from build123d import *

# Parameters (mm, degrees)
SKETCH1_R           = 15.875
BOSS_EXTRUDE1_DEPTH = 12.7
CUT_EXTRUDE1_DEPTH  = 13.7
SKETCH3_R           = 15.875
BOSS_EXTRUDE2_DEPTH = 2.54
SKETCH4_R           = 15.08125
CUT_EXTRUDE2_DEPTH  = 2.54


with BuildPart() as part:
    # Sketch1 → Boss-Extrude1 (new body)
    with BuildSketch(Plane(origin=(0, 0, 0), x_dir=(1, 0, 0), z_dir=(0, 1, 0))):
        Circle(SKETCH1_R)
    extrude(amount=BOSS_EXTRUDE1_DEPTH)

    # Sketch2 → Cut-Extrude1 (cut, through all)
    with BuildSketch(Plane(origin=(0, 12.7, 0), x_dir=(1, 0, 0), z_dir=(0, 1, 0))):
        Polygon((-9.38920922, -5.728023239), (0.266009029, -10.995305325), (9.655218248, -5.267282086), (9.38920922, 5.728023239), (-0.266009029, 10.995305325), (-9.655218248, 5.267282086), align=None)
        Polygon((-5.267282086, -9.655218248), (5.728023239, -9.38920922), (10.995305325, 0.266009029), (5.267282086, 9.655218248), (-5.728023239, 9.38920922), (-10.995305325, -0.266009029), align=None)
        Polygon((-7.13938722, 6.802101287), (-2.781840057, 9.460486124), (-5.728023239, 9.38920922), align=None)
        Polygon((-9.583941344, 2.321098904), (-7.13938722, 6.802101287), (-9.655218248, 5.267282086), align=None)
        Polygon((-10.995305325, -0.266009029), (-9.460486124, -2.781840057), (-9.583941344, 2.321098904), align=None)
        Polygon((-9.38920922, -5.728023239), (-6.802101287, -7.13938722), (-9.460486124, -2.781840057), align=None)
        Polygon((-5.267282086, -9.655218248), (-2.321098904, -9.583941344), (-6.802101287, -7.13938722), align=None)
        Polygon((0.266009029, -10.995305325), (2.781840057, -9.460486124), (-2.321098904, -9.583941344), align=None)
        Polygon((5.728023239, -9.38920922), (7.13938722, -6.802101287), (2.781840057, -9.460486124), align=None)
        Polygon((7.13938722, -6.802101287), (9.655218248, -5.267282086), (9.583941344, -2.321098904), align=None)
        Polygon((9.460486124, 2.781840057), (9.583941344, -2.321098904), (10.995305325, 0.266009029), align=None)
        Polygon((6.802101287, 7.13938722), (9.460486124, 2.781840057), (9.38920922, 5.728023239), align=None)
        Polygon((2.321098904, 9.583941344), (6.802101287, 7.13938722), (5.267282086, 9.655218248), align=None)
        Polygon((-2.781840057, 9.460486124), (2.321098904, 9.583941344), (-0.266009029, 10.995305325), align=None)
    extrude(amount=-CUT_EXTRUDE1_DEPTH, mode=Mode.SUBTRACT)

    # Sketch3 → Boss-Extrude2 (add)
    with BuildSketch(Plane.XZ):
        Circle(SKETCH3_R)
    extrude(amount=BOSS_EXTRUDE2_DEPTH)

    # Sketch4 → Cut-Extrude2 (cut)
    with BuildSketch(Plane.XZ.offset(2.54)):
        Circle(SKETCH4_R)
    extrude(amount=-CUT_EXTRUDE2_DEPTH, mode=Mode.SUBTRACT)


solid = part.part
Build history of the part. All positions in model axes, mm. A direction names the side the tool comes from. Give positions to 0.01 mm unless a question says otherwise; leave off trailing zeros. Loops run counter-clockwise (first coordinate to the right, second up) from the corner with the lowest first, then second, coordinate; pieces in that order, holes last. Notation, with made-up numbers: (33, 33.25) -> (72, 33.25) arc R14 ccw to (72, 58.25) -> close; hole circle Ø4 at (19, 22). An arc over 180 degrees is marked (long way). Answer in a Markdown table with one row per item.
Item 1: Slice it at B-B on z = -4. Write the cut outline in (x, y), plus the area to 3 significant figures.
Findings below:
| item | result |
|---|---|
| outline | (-15.36, -2.54) -> (-14.54, -2.54) -> (-14.54, 0) -> (-9.62, 0) -> (-9.62, 12.7) -> (-15.36, 12.7) -> close; (9.43, 0) -> (14.54, 0) -> (14.54, -2.54) -> (15.36, -2.54) -> (15.36, 12.7) -> (9.43, 12.7) -> close |
| area | 152 mm² |
Item 2: Mould opens along Z. For faces 1 (the flat face through (1.046, 6.439, -10.28)), 2 (the cylindrical face through (-3.441, 5.187, -15.497)), 3 (the flat face through (-7.3, 12.7, -7.3)) say: pulls with the +Z half, pulls with the -Z half, needs draft (parallel to the pull), parting line crosses it, or undercut.
Findings below:
| item | result |
|---|---|
| face 1 | undercut |
| face 2 | parting line crosses it |
| face 3 | needs draft |
Item 3: Slice it at A-A on y = 9.5. Write the cut outline in (x, z) (3 decimals), plus the area to 3 significant figures.
Findings below:
| item | result |
|---|---|
| outline | circle Ø31.75 at (0, 0); hole (-10.995, 0.266) -> (-9.584, -2.321) -> (-9.655, -5.267) -> (-7.139, -6.802) -> (-5.728, -9.389) -> (-2.782, -9.46) -> (-0.266, -10.995) -> (2.321, -9.584) -> (5.267, -9.655) -> (6.802, -7.139) -> (9.389, -5.728) -> (9.46, -2.782) -> (10.995, -0.266) -> (9.584, 2.321) -> (9.655, 5.267) -> (7.139, 6.802) -> (5.728, 9.389) -> (2.782, 9.46) -> (0.266, 10.995) -> (-2.321, 9.584) -> (-5.267, 9.655) -> (-6.802, 7.139) -> (-9.389, 5.728) -> (-9.46, 2.782) -> close |
| area | 455 mm² |
Item 4: Tool access for faces 4 (the flat face through (-8.38, 6.439, -6.045)), 5 (the flat face through (14, -2.54, -6)), 6 (the flat face through (3, 0, -10)): list every direction of +Z, -Z, +X, -X, +Y, -Y with a clear straight run to the whole face (end or side of a thin tool).
Findings below:
| item | result |
|---|---|
| face 4 | +Y, -Y |
| face 5 | +Z, -Z, +X, -X, -Y |
| face 6 | -Y |
Item 5: Flat gauge pins, fed straight in: P1, Ø1, axis at y = 6.5, z = 2.5, coming from the +X side; P2, Ø8, axis at y = 7.5, z = 11, coming from the +X side; P3, Ø1.5, axis at x = -3, y = 2.5, coming from the +Z side. Where does each tip first touch, or does it go through?
Findings below:
| item | result |
|---|---|
| P1 | stops at x = 15.75 |
| P2 | stops at x = 14.25 |
| P3 | stops at z = 15.71 |
Item 6: Slice it at C-C on z = 1. Write the cut outline in (x, y), plus the area to 3 significant figures.
Findings below:
| item | result |
|---|---|
| outline | (-15.84, -2.54) -> (-15.05, -2.54) -> (-15.05, 0) -> (-10.55, 0) -> (-10.55, 12.7) -> (-15.84, 12.7) -> close; (10.3, 0) -> (15.05, 0) -> (15.05, -2.54) -> (15.84, -2.54) -> (15.84, 12.7) -> (10.3, 12.7) -> close |
| area | 142 mm² |
Item 7: Slice it at D-D on z = 13.5. Write the cut outline in (x, y).
Findings below:
| item | result |
|---|---|
| outline | (-8.35, -2.54) -> (-6.72, -2.54) -> (-6.72, 0) -> (6.72, 0) -> (6.72, -2.54) -> (8.35, -2.54) -> (8.35, 12.7) -> (-8.35, 12.7) -> close |
Item 8: Probe line 1 along Z through (x, y) = (0, -1.05) (3 decimals); line 2 along Y through (x, z) = (11.5, 7.5); line 3 along X through (y, z) = (11.75, 0.5). List the from-to ranges inside material, lowest first. Write a range as [from, to].
Findings below:
| item | result |
|---|---|
| line 1 | z = [-15.875, -15.081], [15.081, 15.875] |
| line 2 | y = [0, 12.7] |
| line 3 | x = [-15.87, -10.85], [10.58, 15.87] |
